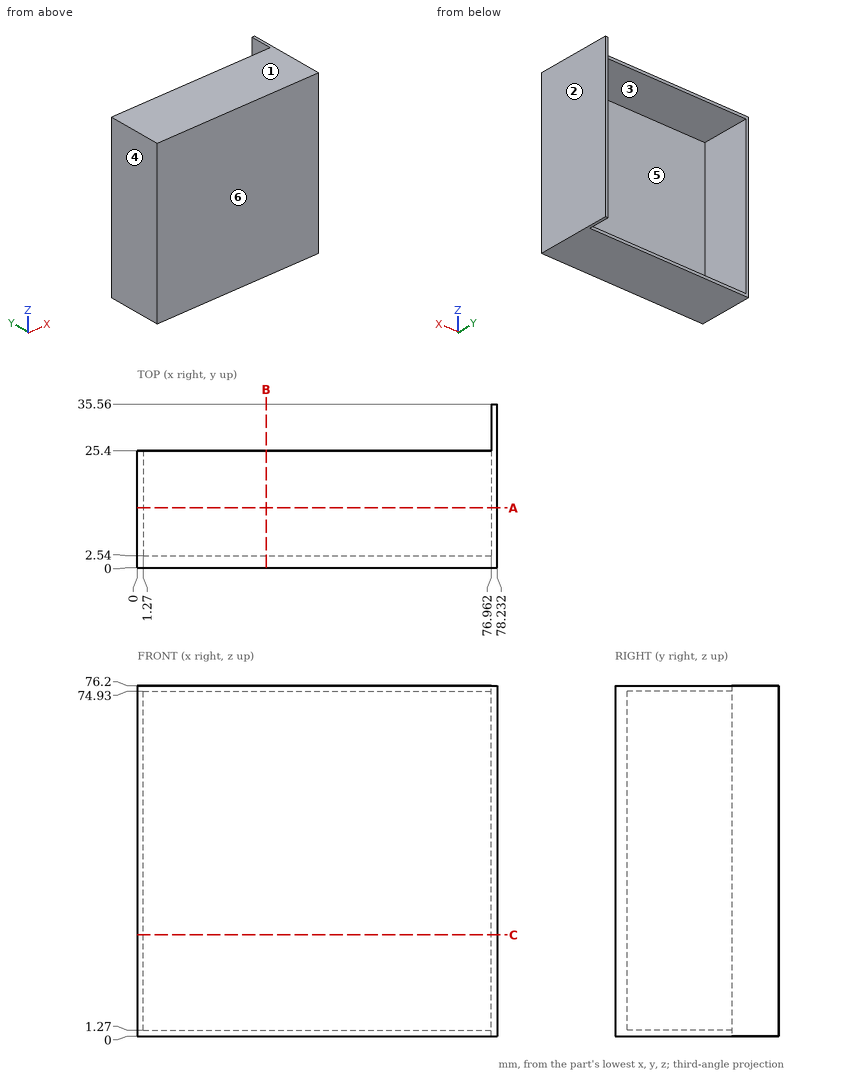
Here's the drawing with two shaded views (mm, measured from the low corner). I have some questions. A direction names the side the tool comes from. Round coordinates to 2 decimals unless told otherwise and drop trailing zeros. Write each loop counter-clockwise with the first axis right and the second up, starting at its lowest first coordinate (ties: lowest second). Pieces come first, ordered by that corner, then holes. Notation, with made-up numbers: M 26,16.5 L 58,16.5 A17 cw 58,32.5 Z; hole C -3,41 d4. An arc over 180 degrees is marked long. Use CSV: the item, a comma, the result in double quotes.
(1) Imagine slicing it at B-B (x = 28). Write out the boundary of the cut face in (y, z), plus the area to 3 significant figures.
Check values:
outline,"M 0,0 L 25.4,0 L 25.4,1.27 L 2.54,1.27 L 2.54,74.93 L 25.4,74.93 L 25.4,76.2 L 0,76.2 Z"
area,"252 mm^2"
(2) Imagine slicing it at C-C (z = 22). Write out the boundary of the cut face in (x, y), plus the area to 3 significant figures.
Check values:
outline,"M 0,0 L 78.23,0 L 78.23,35.56 L 76.96,35.56 L 76.96,2.54 L 1.27,2.54 L 1.27,25.4 L 0,25.4 Z"
area,"270 mm^2"
(3) Imagine slicing it at A-A (y = 13). Write out the boundary of the cut face in (x, z).
Check values:
outline,"M 0,0 L 78.23,0 L 78.23,76.2 L 0,76.2 Z; hole M 1.27,1.27 L 76.96,1.27 L 76.96,74.93 L 1.27,74.93 Z"
(4) On a 3-axis mill with a long thin cutter (end or side, diameter ignored), from which of +Z, -Z, +X, -X, +Y, -Y can I reach the whole of each face in a straight line? I mean the marked faces 5 and 6. Say none if no direction works.
Check values:
face 5,"+Y"
face 6,"+Z, -Z, +X, -X, -Y"
(5) I'm going to push flat-ended pins straight in: pin 1 (4 mm diameter, centred on x = 30.5, y = 6, fed in from -Z); pin 2 (23 mm diameter, centred on x = 39, z = 26.5, fed in from +Y). Where does each tip first touch, or does it pass through?
Check values:
pin 1,"z = 0"
pin 2,"y = 2.54"
(6) We'd pull the mould along X, two halves only. Please class the marked faces 1, 2, 3 and 4: +X half, -X half, draft (parallel to the pull), parting line (faces both ways), or undercut.
Check values:
face 1,"draft"
face 2,"+X half"
face 3,"undercut"
face 4,"-X half"
(7) I need wall thicknesses on line 1 along X through (y, z) = (12.5, 28.5); line 2 along Z through (x, y) = (12, 4); line 3 along Y through (x, z) = (66.5, 18). Which ranges of each line are inside material? Lowest first, please.
Check values:
line 1,"0 to 1.27, 76.96 to 78.23"
line 2,"0 to 1.27, 74.93 to 76.2"
line 3,"0 to 2.54"
